from build123d import *

# Parameters (mm, degrees)
SKETCH1_R           = 0.375
BOSS_EXTRUDE1_DEPTH = 0.7874
BOSS_EXTRUDE2_DEPTH = 2.3
FILLET1_R           = 0.5
SKETCH3_R           = 0.508
CUT_EXTRUDE1_DEPTH  = 0.7874


with BuildPart() as part:
    # Sketch1 → Boss-Extrude1 (new body)
    with BuildSketch(Plane(origin=(0, 0, 0), x_dir=(1, 0, 0), z_dir=(0, 1, 0))):
        Polygon((-1, 8.25), (-1, 10.1), (1, 10.1), (1, 8.25), (6.65, 8.25), (6.65, -0.858517924), (8.5, -0.858517924), (8.5, -2.858517924), (6.65, -2.858517924), (6.65, -8.25), (-6.65, -8.25), (-6.65, -2.858517924), (-8.5, -2.858517924), (-8.5, -0.858517924), (-6.65, -0.858517924), (-6.65, 8.25), align=None)
        with Locations(Location((-7.5, -1.858517924, 0), (0, 0, 270))):
            Circle(SKETCH1_R, mode=Mode.SUBTRACT)
        with Locations(Location((7.5, -1.858517924, 0), (0, 0, 270))):
            Circle(SKETCH1_R, mode=Mode.SUBTRACT)
        with Locations(Location((0, 9.141482076, 0), (0, 0, 270))):
            Circle(SKETCH1_R, mode=Mode.SUBTRACT)
    extrude(amount=BOSS_EXTRUDE1_DEPTH)

    # Sketch2 → Boss-Extrude2 (add)
    with BuildSketch(Plane(origin=(0, 0.7874, 0), x_dir=(1, 0, 0), z_dir=(0, 1, 0))):
        with BuildLine():
            Line((5.65, 7.55), (-5.65, 7.55))
            ThreePointArc((-5.65, 7.55), (-5.862132034, 7.462132034), (-5.95, 7.25))
            Line((-5.95, 7.25), (-5.95, -4.05))
            ThreePointArc((-5.95, -4.05), (-5.862132034, -4.262132034), (-5.65, -4.35))
            Line((-5.65, -4.35), (5.65, -4.35))
            ThreePointArc((5.65, -4.35), (5.862132034, -4.262132034), (5.95, -4.05))
            Line((5.95, -4.05), (5.95, 7.25))
            ThreePointArc((5.95, 7.25), (5.862132034, 7.462132034), (5.65, 7.55))
        make_face()
    extrude(amount=BOSS_EXTRUDE2_DEPTH)

    # Fillet1
    fillet1_edges = [part.edges().sort_by_distance(p)[0] for p in [
        (-6.65, 0.3937, 2.858517924),
        (-8.5, 0.3937, 2.858517924),
        (-8.5, 0.3937, 0.858517924),
        (-6.65, 0.3937, 0.858517924),
        (-6.65, 0.3937, -8.25),
        (-1, 0.3937, -8.25),
        (-1, 0.3937, -10.1),
        (1, 0.3937, -10.1),
        (1, 0.3937, -8.25),
        (6.65, 0.3937, -8.25),
        (6.65, 0.3937, 0.858517924),
        (8.5, 0.3937, 0.858517924),
        (8.5, 0.3937, 2.858517924),
        (6.65, 0.3937, 2.858517924),
        (6.65, 0.3937, 8.25),
        (-6.65, 0.3937, 8.25),
    ]]
    fillet(fillet1_edges, radius=FILLET1_R)

    # Sketch3 → Cut-Extrude1 (cut)
    with BuildSketch(Plane(origin=(0, 0.7874, 0), x_dir=(1, 0, 0), z_dir=(0, 1, 0))):
        with Locations(Location((0, -5.76619869, 0), (0, 0, 270))):
            Circle(SKETCH3_R)
        with Locations(Location((0, -7.03619869, 0), (0, 0, 270))):
            Circle(SKETCH3_R)
    extrude(amount=-CUT_EXTRUDE1_DEPTH, mode=Mode.SUBTRACT)


solid = part.part
The listing builds one solid part. Answer for the finished solid, in the listing's coordinates (mm). A direction names the side the tool comes from. Coordinates: 2 decimals unless noted, no trailing zeros. Loops run counter-clockwise (first coordinate to the right, second up) from the corner with the lowest first, then second, coordinate; pieces in that order, holes last.
1) Flat-ended cylindrical pins translate along their axes: pin 1 Ø1.5 at (x, z) = (-5, -6.5) entering from -Y; pin 2 Ø0.6 at (y, z) = (0.5, -3) entering from +X; pin 3 Ø0.9 at (x, y) = (7.5, 0) entering from +Z; pin 4 Ø1.8 at (y, z) = (2, -3) entering from +X. Find the tip coordinate at first contact, or state that the pin passes through.
2) Determine the mould class of faces 6 (the face through (-5.95, 2, -2)), 7 (the face through (0, 2, 4.35)), 8 (the face through (0.15, 0.4, 7.52)), 9 (the face through (0.15, 0.4, 6.25)) for opening direction X: pulls with the +X half, pulls with the -X half, needs draft (parallel to the pull), parting line crosses it, or undercut.
3) Find section A-A on x = 0. Write down the section's boundary in (y, z), then the cut area to 3 significant figures.
4) Find section B-B on y = 1.2. Write down the section's boundary in (x, z), then the cut area to 3 significant figures.
5) A tool of negligible diameter and unlimited length cuts with its end or side. For faces 1 (the face through (0, 2, -7.55)), 2 (the face through (0, 3.087, -2)), 3 (the face through (5.95, 2, -2)), 4 (the face through (0.7, 0.787, 4.5)), 5 (the face through (0, 0, -1)), from which of +Z, -Z, +X, -X, +Y, -Y can it reach the whole face along a straight path? Write none if from no direction.
6) Find section C-C on z = -2.5. Write down the section's boundary in (x, y).
7) Find the intervals of material crossed by L1, parallel to X at y = 2.65, z = -1.5; L2, parallel to Z at x = 4, y = 1.7, in increasing order.
8) Find section D-D on x = 7.5. Write down the section's boundary in (y, z).
Values:
1. pin 1: stops at y = 0
1. pin 2: stops at x = 6.65
1. pin 3: stops at z = 2.87
1. pin 4: stops at x = 5.95
2. face 6: pulls with the -X half
2. face 7: needs draft
2. face 8: undercut
2. face 9: undercut
3. outline: (0, -10.1) - (0.79, -10.1) - (0.79, -9.52) - (0, -9.52) - close; (0, -8.77) - (0.79, -8.77) - (0.79, -7.55) - (3.09, -7.55) - (3.09, 4.35) - (0.79, 4.35) - (0.79, 5.26) - (0, 5.26) - close; (0, 6.27) - (0.79, 6.27) - (0.79, 6.53) - (0, 6.53) - close; (0, 7.54) - (0.79, 7.54) - (0.79, 8.25) - (0, 8.25) - close
3. area: 39.6 mm2
4. outline: (-5.95, -7.25) arc R0.3 ccw to (-5.65, -7.55) - (5.65, -7.55) arc R0.3 ccw to (5.95, -7.25) - (5.95, 4.05) arc R0.3 ccw to (5.65, 4.35) - (-5.65, 4.35) arc R0.3 ccw to (-5.95, 4.05) - close
4. area: 142 mm2
5. face 1: -Z, +X, -X, +Y
5. face 2: +Z, -Z, +X, -X, +Y
5. face 3: +Z, -Z, +X, +Y
5. face 4: +Y
5. face 5: +Z, -Z, +X, -X, -Y
6. outline: (-6.65, 0) - (6.65, 0) - (6.65, 0.79) - (5.95, 0.79) - (5.95, 3.09) - (-5.95, 3.09) - (-5.95, 0.79) - (-6.65, 0.79) - close
7. L1: x = -5.95 to 5.95
7. L2: z = -7.55 to 4.35
8. outline: (0, 0.86) - (0.79, 0.86) - (0.79, 1.48) - (0, 1.48) - close; (0, 2.23) - (0.79, 2.23) - (0.79, 2.86) - (0, 2.86) - close
